Could you check a few things on this model? Use its own coordinates, in mm. Coordinates: 2 decimals unless noted, no trailing zeros. Write each loop counter-clockwise with the first axis right and the second up, starting at its lowest first coordinate (ties: lowest second). Pieces come first, ordered by that corner, then holes. Notation, with made-up numbers: M 23,17 L 41,17 A12 ccw 41,30 Z; hole C 31.25,72 d9. An arc over 180 degrees is marked long. Answer as CSV lines item,"result". Start each with the question number.
Item 1: We'd pull the mould along Z, two halves only. Please class faces 1 (the cylindrical face through (-0.275, 1.565, -3.523)), 2 (the cylindrical face through (-57.564, 1.565, -4.276)), 3 (the flat face through (-1, 2, -15.875)), 4 (the flat face through (-1, 0, -2)): +Z half, -Z half, draft (parallel to the pull), parting line (faces both ways), or undercut.
Item 2: If I drill on line 1 along X through (y, z) = (1.35, 8); line 2 along X through (y, z) = (2.85, 8.25); line 3 along Z through (x, y) = (-0.5, 0.25) (3 decimals), over which ranges is the centre line in solid material (lowest first)? Write a range as [from, to].
Item 3: Suppose I cut it at A-A, the plane x = 0. Write out the boundary of the cut face in (y, z) (1 decimal).
```python
from build123d import *

# Parameters (mm, degrees)
SKETCH1_W           = 127
SKETCH1_H           = 25.4
SKETCH1_R           = 1.27
SKETCH1_H_2         = 3.175
BOSS_EXTRUDE1_DEPTH = 3.175


with BuildPart() as part:
    # Sketch1 → Boss-Extrude1 (new body)
    with BuildSketch(Plane(origin=(0, 0, 0), x_dir=(1, 0, 0), z_dir=(0, 1, 0))):
        Rectangle(SKETCH1_W, SKETCH1_H)
        with Locations((58.7375, -7.9375)):
            Circle(SKETCH1_R, mode=Mode.SUBTRACT)
        with Locations((0, -7.9375)):
            Circle(SKETCH1_R, mode=Mode.SUBTRACT)
        with Locations((-58.7375, -7.9375)):
            Circle(SKETCH1_R, mode=Mode.SUBTRACT)
        with Locations((58.7375, 4.7625)):
            Circle(SKETCH1_R, mode=Mode.SUBTRACT)
        with Locations((0, 4.7625)):
            Circle(SKETCH1_R, mode=Mode.SUBTRACT)
        with Locations((-58.7375, 4.7625)):
            Circle(SKETCH1_R, mode=Mode.SUBTRACT)
        with Locations((0, 14.2875)):
            Rectangle(SKETCH1_W, SKETCH1_H_2)
    extrude(amount=BOSS_EXTRUDE1_DEPTH)


solid = part.part
```
Ans:
1,face 1,"undercut"
1,face 2,"undercut"
1,face 3,"-Z half"
1,face 4,"draft"
2,line 1,"x = [-63.5, -60.01], [-57.47, -1.27], [1.27, 57.47], [60.01, 63.5]"
2,line 2,"x = [-63.5, -59.97], [-57.51, -1.23], [1.23, 57.51], [59.97, 63.5]"
2,line 3,"z = [-15.875, -5.93], [-3.595, 6.77], [9.105, 12.7]"
3,outline,"M 0,-15.9 L 3.2,-15.9 L 3.2,-6 L 0,-6 Z; M 0,-3.5 L 3.2,-3.5 L 3.2,6.7 L 0,6.7 Z; M 0,9.2 L 3.2,9.2 L 3.2,12.7 L 0,12.7 Z"
